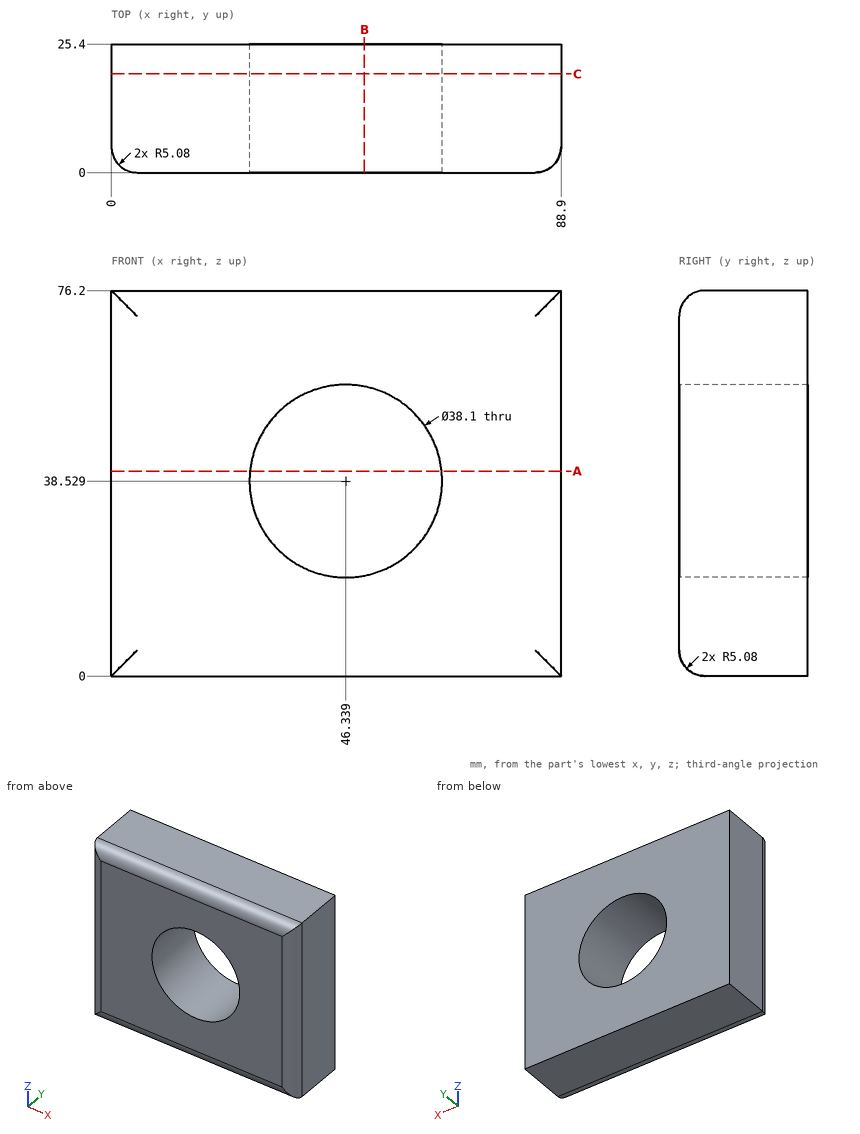
Source: three-view drawing plus pictorial views. Frame: mm from the lowest corner of the part. Round coordinates to 2 decimals unless told otherwise and drop trailing zeros. Loops run counter-clockwise (first coordinate to the right, second up) from the corner with the lowest first, then second, coordinate; pieces in that order, holes last. Notation, with made-up numbers: (-1.5, -21.5) - (36.5, -21.5) arc R22 ccw to (36.5, 14.5) - close; hole circle Ø9 at (37, -18.5). An arc over 180 degrees is marked (long way). Write item = value, one per line. Start each with the question number.
Item 1: Section query B-B on x = 50. Output: boundary loops of the cut face in (y, z) (1 decimal).
Item 2: Section query A-A on z = 40.5. Output: boundary loops of the cut face in (x, y), plus the area to 3 significant figures.
Item 3: Material intervals for line 1 (X direction, y = 18, z = 28) (1 decimal); line 2 (X direction, y = 21.5, z = 55.5) (1 decimal); line 3 (Z direction, x = 32.5, y = 12), sorted ascending.
Item 4: Section query C-C on y = 19.5. Output: boundary loops of the cut face in (x, z).
Item 5: First-contact query: pin 1 Ø6 at (x, z) = (9, 24.5) entering from -Y; pin 2 Ø2 at (y, z) = (2.5, 22.5) entering from +X. Flat tips, straight axial feed; report the tip coordinate or a pass-through.
Results list:
q1.outline = (0, 5.1) arc R5.1 ccw to (5.1, 0) - (25.4, 0) - (25.4, 19.8) - (0, 19.8) - close; (0, 57.2) - (25.4, 57.2) - (25.4, 76.2) - (5.1, 76.2) arc R5.1 ccw to (0, 71.1) - close
q2.outline = (0, 5.08) arc R5.08 ccw to (5.08, 0) - (27.39, 0) - (27.39, 25.4) - (0, 25.4) - close; (65.29, 0) - (83.82, 0) arc R5.08 ccw to (88.9, 5.08) - (88.9, 25.4) - (65.29, 25.4) - close
q2.area = 1,280 mm²
q3.line_1 = 0 to 30.5, 62.2 to 88.9
q3.line_2 = 0 to 37.7, 55 to 88.9
q3.line_3 = 0 to 25.44, 51.62 to 76.2
q4.outline = (0, 0) - (88.9, 0) - (88.9, 76.2) - (0, 76.2) - close; hole circle Ø38.1 at (46.34, 38.53)
q5.pin_1 = 0
q5.pin_2 = 88.65
